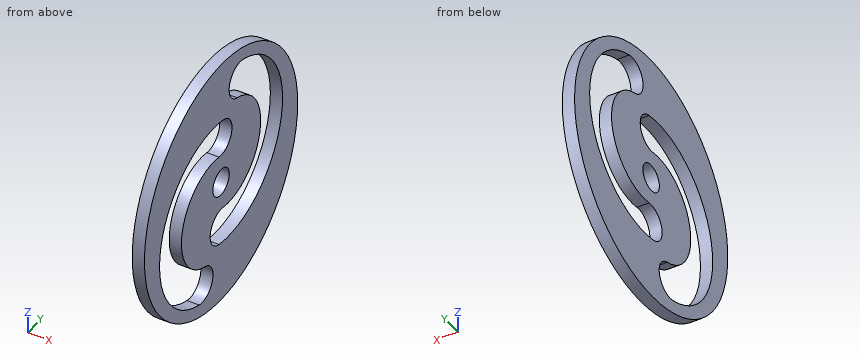
```python
from build123d import *

# Parameters (mm, degrees)
F0_R     = 21
F0_R_2   = 2.25
F1_DEPTH = 2


with BuildPart() as f1:
    # F0 (on Right) → F1 (new body)
    with BuildSketch(Plane.YZ):
        Circle(F0_R)
        with BuildLine():
            ThreePointArc((-4.423462, -12.115904), (-2.310416, -15.794904), (-5.989415, -17.90795))
            ThreePointArc((-5.989415, -17.90795), (-16.493635, -0.432608), (0.55056, 10.757637))
            ThreePointArc((0.55056, 10.757637), (2.949048, 7.258029), (-0.55056, 4.859542))
            ThreePointArc((-0.55056, 4.859542), (-10.643946, -1.767199), (-4.423462, -12.115904))
        make_face(mode=Mode.SUBTRACT)
        Circle(F0_R_2, mode=Mode.SUBTRACT)
        with BuildLine():
            ThreePointArc((-0.55056, -10.757637), (-2.949048, -7.258029), (0.55056, -4.859542))
            ThreePointArc((0.55056, -4.859542), (10.643946, 1.767199), (4.423462, 12.115904))
            ThreePointArc((4.423462, 12.115904), (2.310416, 15.794904), (5.989415, 17.90795))
            ThreePointArc((5.989415, 17.90795), (16.493635, 0.432608), (-0.55056, -10.757637))
        make_face(mode=Mode.SUBTRACT)
    extrude(amount=F1_DEPTH)


solid = f1.part
```
CAD build for the part. Positions are in the model's coordinates, mm. Give positions to 0.01 mm unless a question says otherwise; leave off trailing zeros. Loops run counter-clockwise (first coordinate to the right, second up) from the corner with the lowest first, then second, coordinate; pieces in that order, holes last. Notation, with made-up numbers: (-33, 57.5) -> (8, 57.5) arc R14 cw to (8, 84.5) -> close; hole circle Ø11 at (58, -40). An arc over 180 degrees is marked (long way). Use a Markdown table: item, result.
1. Slice it at C-C (z = 0). List the corners of the cut face in (x, y), plus the area to 3 significant figures.
Check result:
| item | result |
|---|---|
| outline | (0, -21) -> (2, -21) -> (2, -16.39) -> (0, -16.39) -> close; (0, -10.04) -> (2, -10.04) -> (2, -2.25) -> (0, -2.25) -> close; (0, 2.25) -> (2, 2.25) -> (2, 10.04) -> (0, 10.04) -> close; (0, 16.39) -> (2, 16.39) -> (2, 21) -> (0, 21) -> close |
| area | 49.6 mm^2 |
2. Slice it at A-A (y = 15.5). List the corners of the cut face in (x, z).
Check result:
| item | result |
|---|---|
| outline | (0, -14.17) -> (2, -14.17) -> (2, -2.48) -> (0, -2.48) -> close; (0, 9.89) -> (2, 9.89) -> (2, 14.17) -> (0, 14.17) -> close |
3. Wall check: L1, parallel to Z at x = 0.7, y = 6; L2, parallel to Z at x = 1.35, y = 0; L3, parallel to Z at x = 0.1, y = 9. Give the ranges that are in metal, low to high. Write a range as [from, to].
Check result:
| item | result |
|---|---|
| L1 | z = [-20.12, -10.49], [-4.11, 11.52], [17.91, 20.12] |
| L2 | z = [-21, -10.85], [-4.81, -2.25], [2.25, 4.81], [10.85, 21] |
| L3 | z = [-18.97, -9.32], [-1.68, 9.09], [16.73, 18.97] |
4. Slice it at D-D (y = 0). List the corners of the cut face in (x, z), plus the area to 3 significant figures.
Check result:
| item | result |
|---|---|
| outline | (0, -21) -> (2, -21) -> (2, -10.85) -> (0, -10.85) -> close; (0, -4.81) -> (2, -4.81) -> (2, -2.25) -> (0, -2.25) -> close; (0, 2.25) -> (2, 2.25) -> (2, 4.81) -> (0, 4.81) -> close; (0, 10.85) -> (2, 10.85) -> (2, 21) -> (0, 21) -> close |
| area | 50.8 mm^2 |
5. Slice it at B-B (z = -11.5). List the corners of the cut face in (x, y).
Check result:
| item | result |
|---|---|
| outline | (0, -17.57) -> (2, -17.57) -> (2, -14.63) -> (0, -14.63) -> close; (0, -6.04) -> (2, -6.04) -> (2, 17.57) -> (0, 17.57) -> close |
